from build123d import *

# Parameters (mm, degrees)
SKETCH1_W            = 110
SKETCH1_H            = 58
BOSS_EXTRUDE1_DEPTH  = 4
SKETCH2_R            = 3.398974158
SKETCH2_R_2          = 3.407761536
SKETCH2_R_3          = 1.902710934
SKETCH2_R_4          = 2.384440654
BOSS_EXTRUDE2_DEPTH  = 1.6
BOSS_EXTRUDE3_DEPTH  = 6.2
SKETCH4_R            = 2.45
SKETCH4_R_2          = 1.95
SKETCH4_R_3          = 1.9
SKETCH4_R_4          = 1.2
BOSS_EXTRUDE4_DEPTH  = 4
BOSS_EXTRUDE5_DEPTH  = 1.6
BOSS_EXTRUDE7_DEPTH  = 2
SKETCH10_W           = 9.685953709
SKETCH10_H           = 3.389605022
CUT_EXTRUDE1_DEPTH   = 5
SKETCH11_W           = 9.457855186
SKETCH11_H           = 3.19445865
CUT_EXTRUDE2_DEPTH   = 5
SKETCH12_W           = 7.571734997
SKETCH12_H           = 3.389605022
CUT_EXTRUDE3_DEPTH   = 5
SKETCH13_W           = 8.877658174
SKETCH13_H           = 3.389605022
CUT_EXTRUDE4_DEPTH   = 5
BOSS_EXTRUDE11_DEPTH = 2
SKETCH15_W           = 2.328463334
SKETCH15_H           = 10.356170305
SKETCH15_W_2         = 2.062506364
SKETCH15_H_2         = 9.72645826
SKETCH15_W_3         = 2.09471635
SKETCH15_H_3         = 7.99735701
SKETCH15_W_4         = 2.398553281
CUT_EXTRUDE5_DEPTH   = 10
SKETCH16_R           = 1.5
CUT_EXTRUDE9_DEPTH   = 5


with BuildPart() as part:
    # Sketch1 → Boss-Extrude1 (new body)
    with BuildSketch(Plane(origin=(0, 0, 0), x_dir=(1, 0, 0), z_dir=(0, 1, 0))):
        Rectangle(SKETCH1_W, SKETCH1_H)
    extrude(amount=BOSS_EXTRUDE1_DEPTH)

    # Sketch2 → Boss-Extrude2 (add)
    with BuildSketch(Plane(origin=(0, 4, 0), x_dir=(1, 0, 0), z_dir=(0, 1, 0))):
        Polygon((46.346119795, 25.541263413), (55, 25.541263413), (55, 29), (-54.994341331, 29), (-54.994341331, 25.541263413), (-45.986579734, 25.541263413), (-45.986579734, 18.10232226), (-45.986579734, 17.980527053), (-45.986579734, 16.083408227), (-45.088264615, 15.185093108), (-42.202263878, 15.185093108), (-41.564501972, 15.822855015), (-41.564501972, 18.10232226), (-41.564501972, 25.541263413), (40.304214547, 25.541263413), (41.797555033, 20.604809993), (41.797555033, 16.117567037), (42.441634266, 15.185093108), (45.678891317, 15.185093108), (46.346119795, 16.117567037), align=None)
        with Locations(Location((-13.880988948, 17.14491543, 0), (0, 0, 270))):
            Circle(SKETCH2_R)
        with Locations(Location((20.080301926, 13.55493457, 0), (0, 0, 270))):
            Circle(SKETCH2_R_2)
        with Locations(Location((20.58969132, -10.683370151, 0), (0, 0, 270))):
            Circle(SKETCH2_R_3)
        with Locations(Location((-19.024959871, -10.704463559, 0), (0, 0, 270))):
            Circle(SKETCH2_R_4)
        Polygon((-55, -25.732689432), (-55, -29), (55, -29), (55, -25.732689432), (46.191771323, -25.732689432), (46.191771323, -17.749211072), (41.797555033, -17.720096968), (41.797555033, -25.732689432), (-41.564501972, -25.732689432), (-41.564501972, -19.505766322), (-41.564501972, -16.046735723), (-45.837931694, -16.046735723), (-45.837931694, -19.079806126), (-45.837931694, -25.732689432), (-46.135227773, -25.732689432), align=None)
    extrude(amount=BOSS_EXTRUDE2_DEPTH)

    # Sketch2 → Boss-Extrude3 (add)
    with BuildSketch(Plane(origin=(0, 4, 0), x_dir=(1, 0, 0), z_dir=(0, 1, 0))):
        Polygon((46.346119795, 25.541263413), (55, 25.541263413), (55, 29), (-54.994341331, 29), (-54.994341331, 25.541263413), (-45.986579734, 25.541263413), (-45.986579734, 18.10232226), (-45.986579734, 17.980527053), (-45.986579734, 16.083408227), (-45.088264615, 15.185093108), (-42.202263878, 15.185093108), (-41.564501972, 15.822855015), (-41.564501972, 18.10232226), (-41.564501972, 25.541263413), (40.304214547, 25.541263413), (41.797555033, 20.604809993), (41.797555033, 16.117567037), (42.441634266, 15.185093108), (45.678891317, 15.185093108), (46.346119795, 16.117567037), align=None)
        with Locations(Location((-13.880988948, 17.14491543, 0), (0, 0, 270))):
            Circle(SKETCH2_R)
        with Locations(Location((20.080301926, 13.55493457, 0), (0, 0, 270))):
            Circle(SKETCH2_R_2)
        with Locations(Location((20.58969132, -10.683370151, 0), (0, 0, 270))):
            Circle(SKETCH2_R_3)
        with Locations(Location((-19.024959871, -10.704463559, 0), (0, 0, 270))):
            Circle(SKETCH2_R_4)
        Polygon((-55, -25.732689432), (-55, -29), (55, -29), (55, -25.732689432), (46.191771323, -25.732689432), (46.191771323, -17.749211072), (41.797555033, -17.720096968), (41.797555033, -25.732689432), (-41.564501972, -25.732689432), (-41.564501972, -19.505766322), (-41.564501972, -16.046735723), (-45.837931694, -16.046735723), (-45.837931694, -19.079806126), (-45.837931694, -25.732689432), (-46.135227773, -25.732689432), align=None)
    extrude(amount=BOSS_EXTRUDE3_DEPTH)

    # Sketch4 → Boss-Extrude4 (add)
    with BuildSketch(Plane(origin=(0, 10.2, 0), x_dir=(1, 0, 0), z_dir=(0, 1, 0))):
        with Locations(Location((-13.880988948, 17.14491543, 0), (0, 0, 270))):
            Circle(SKETCH4_R)
        with Locations(Location((20.080301926, 13.55493457, 0), (0, 0, 270))):
            Circle(SKETCH4_R_2)
        with Locations(Location((20.58969132, -10.683370151, 0), (0, 0, 270))):
            Circle(SKETCH4_R_3)
        with Locations(Location((-19.024959871, -10.704463559, 0), (0, 0, 270))):
            Circle(SKETCH4_R_4)
    extrude(amount=BOSS_EXTRUDE4_DEPTH)

    # Sketch5 → Boss-Extrude5 (add)
    with BuildSketch(Plane(origin=(0, 10.2, 0), x_dir=(1, 0, 0), z_dir=(0, 1, 0))):
        Polygon((-54.994341331, 25.541263413), (-54.994341331, 29), (55, 29), (55, 25.541263413), (46.346119795, 25.541263413), (46.346119795, 16.117567037), (45.678891317, 15.185093108), (42.441634266, 15.185093108), (41.797555033, 16.117567037), (41.797555033, 20.604809993), (40.304214547, 25.541263413), (-41.564501972, 25.541263413), (-41.564501972, 18.624421299), (-45.986579734, 18.624421299), (-45.986579734, 25.541263413), align=None)
        Polygon((-55, -29), (-55, -25.732689432), (-45.837931694, -25.732689432), (-45.837931694, -16.046735723), (-41.564501972, -16.046735723), (-41.564501972, -25.732689432), (41.797555033, -25.732689432), (41.797555033, -17.720096968), (46.191771323, -17.749211072), (46.191771323, -25.732689432), (55, -25.732689432), (55, -29), align=None)
    extrude(amount=BOSS_EXTRUDE5_DEPTH)

    # Sketch8 → Boss-Extrude7 (add)
    with BuildSketch(Plane(origin=(0, 11.8, 0), x_dir=(1, 0, 0), z_dir=(0, 1, 0))):
        Polygon((-45.986579734, 25.541263413), (-54.994341331, 25.541263413), (-54.994341331, 29), (55, 29), (55, 25.541263413), (46.346119795, 25.541263413), (46.346119795, 16.117567037), (45.678891317, 15.185093108), (42.441634266, 15.185093108), (41.797555033, 16.117567037), (41.80446192, 16.117567037), (41.80446192, 20.605491868), (41.797555033, 20.604809993), (40.304214547, 25.541263413), (-41.564501972, 25.541263413), (-41.564501972, 24.347016348), (-41.542415728, 24.347016348), (-41.542415728, 18.624421299), (-45.986579734, 18.624421299), align=None)
        Polygon((-55, -29), (-55, -25.732689432), (-45.837931694, -25.732689432), (-45.837931694, -16.046735723), (-41.564501972, -16.046735723), (-41.553155446, -16.046735723), (-41.553155446, -22.919153082), (-41.564501972, -22.919153082), (-41.564501972, -25.732689432), (41.797555033, -25.732689432), (41.797555033, -23.239047925), (41.783488135, -23.239047925), (41.783488135, -19.482944402), (46.191771323, -19.482944402), (46.191771323, -25.732689432), (55, -25.732689432), (55, -29), align=None)
    extrude(amount=BOSS_EXTRUDE7_DEPTH)

    # Sketch10 → Cut-Extrude1 (cut)
    with BuildSketch(Plane.ZY.offset(45.837931694)):
        with Locations((20.889712577, 7.400343861)):
            Rectangle(SKETCH10_W, SKETCH10_H)
    extrude(amount=-CUT_EXTRUDE1_DEPTH, mode=Mode.SUBTRACT)

    # Sketch11 → Cut-Extrude2 (cut)
    with BuildSketch(Plane.ZY.offset(45.986579734)):
        with Locations((-20.81233582, 7.302770675)):
            Rectangle(SKETCH11_W, SKETCH11_H)
    extrude(amount=-CUT_EXTRUDE2_DEPTH, mode=Mode.SUBTRACT)

    # Sketch12 → Cut-Extrude3 (cut)
    with BuildSketch(Plane(origin=(46.191771323, 0, 0), x_dir=(0, 0, -1), z_dir=(1, 0, 0))):
        with Locations((-21.535078571, 7.400343861)):
            Rectangle(SKETCH12_W, SKETCH12_H)
    extrude(amount=-CUT_EXTRUDE3_DEPTH, mode=Mode.SUBTRACT)

    # Sketch13 → Cut-Extrude4 (cut)
    with BuildSketch(Plane(origin=(46.346119795, 0, 0), x_dir=(0, 0, -1), z_dir=(1, 0, 0))):
        with Locations((20.556396124, 7.400343861)):
            Rectangle(SKETCH13_W, SKETCH13_H)
    extrude(amount=-CUT_EXTRUDE4_DEPTH, mode=Mode.SUBTRACT)

    # Sketch14 → Boss-Extrude11 (add)
    with BuildSketch(Plane(origin=(0, 13.8, 0), x_dir=(1, 0, 0), z_dir=(0, 1, 0))):
        Polygon((-55, -25.732689432), (-55, -29), (55, -29), (55, -25.732689432), (46.191771323, -25.732689432), (46.191771323, -19.482944402), (40.796637058, -19.482944402), (40.796637058, -23.53105864), (41.797555033, -23.53105864), (41.797555033, -25.732689432), (-41.564501972, -25.732689432), (-41.564501972, -22.919153082), (-41.558372671, -22.919153082), (-41.553155446, -20.524286948), (-40.212145481, -20.524286948), (-40.212145481, -16.046735723), (-45.837931694, -16.046735723), (-45.837931694, -25.732689432), align=None)
        Polygon((55, 29), (-54.994341331, 29), (-54.994341331, 25.541263413), (-45.986579734, 25.541263413), (-45.986579734, 18.624421299), (-40.393969825, 18.624421299), (-40.393969825, 22.074882647), (-41.564501972, 22.074882647), (-41.564501972, 25.541263413), (40.304214547, 25.541263413), (41.797555033, 20.604809993), (41.797555033, 18.88036778), (40.93151342, 18.88036778), (40.93151342, 15.577482073), (41.797555033, 15.577482073), (41.797555033, 14.916904931), (46.346119795, 14.916904931), (46.346119795, 25.541263413), (55, 25.541263413), align=None)
    extrude(amount=BOSS_EXTRUDE11_DEPTH)

    # Sketch15 → Cut-Extrude5 (cut)
    with BuildSketch(Plane(origin=(0, 15.8, 0), x_dir=(1, 0, 0), z_dir=(0, 1, 0))):
        with Locations((-44.822348067, 20.36317826)):
            Rectangle(SKETCH15_W, SKETCH15_H)
        with Locations((-44.806678512, -20.909964853)):
            Rectangle(SKETCH15_W_2, SKETCH15_H_2)
        with Locations((45.144413148, -21.734010927)):
            Rectangle(SKETCH15_W_3, SKETCH15_H_3)
        with Locations((45.146843155, 20.36317826)):
            Rectangle(SKETCH15_W_4, SKETCH15_H)
    extrude(amount=-CUT_EXTRUDE5_DEPTH, mode=Mode.SUBTRACT)

    # Sketch16 → Cut-Extrude9 (cut)
    with BuildSketch(Plane(origin=(0, 4, 0), x_dir=(1, 0, 0), z_dir=(0, 1, 0))):
        with Locations(Location((-49.750520398, -21.917426264, 0), (0, 0, 270))):
            Circle(SKETCH16_R)
        with Locations(Location((-49.750520398, 21.99224412, 0), (0, 0, 270))):
            Circle(SKETCH16_R)
        with Locations(Location((50.339499411, -21.917426264, 0), (0, 0, 270))):
            Circle(SKETCH16_R)
        with Locations(Location((50.339499411, 21.99224412, 0), (0, 0, 270))):
            Circle(SKETCH16_R)
    extrude(amount=-CUT_EXTRUDE9_DEPTH, mode=Mode.SUBTRACT)


solid = part.part
The model under review builds one solid part; all positions refer to its coordinate system, in mm. A direction names the side the tool comes from. Round coordinates to 2 decimals unless told otherwise and drop trailing zeros. Loops run counter-clockwise (first coordinate to the right, second up) from the corner with the lowest first, then second, coordinate; pieces in that order, holes last. Notation, with made-up numbers: M 9,83.25 L 57,83.25 A18 ccw 57,103.25 Z; hole C -10.5,33.25 d1. An arc over 180 degrees is marked long. Answer as CSV lines item,"result". Start each with the question number.
Item 1: Consider section B-B (z = -5.5). Write out the cut boundary in (x, y), then the cut area to 3 significant figures.
Item 2: Insertion check: P1, Ø4, axis at x = 22.5, z = 15, coming from the +Y side; P2, Ø0.9, axis at y = 5, z = -21, coming from the -X side; P3, Ø5, axis at y = 12.5, z = 16, coming from the -X side. Each pin has a flat end and moves straight along its axis. Give the tip position at first contact, or say it passes through.
Item 3: Wall thickness on line 1 (Y direction, x = -43, z = -23.5); line 2 (Z direction, x = 50, y = 13.5); line 3 (Y direction, x = 43, z = -18): over which ranges is each line inside the solid? List them lowest first. Write a range as [from, to].
Item 4: Consider section C-C (y = 7.75). State how many separate pieces and enclosed holes the cut face has, then the cut area to 3 significant figures.
Item 5: For faces 4 (the face through (43, 7, -16.118)), 5 (the face through (-17.2, 7.06, -17.88)), 6 (the face through (-42, 7, -16.083)), list the 3-axis set-ups (+Z, -Z, +X, -X, +Y, -Y) from which the entire face can be reached by the end or side of a thin tool; tool diameter is ignored.
Item 6: Mouldability with a two-part tool opening along X and no side actions: class faces 1 (the face through (-12, 10.2, -15)), 2 (the face through (43.948, 12, -20)), 3 (the face through (43, 7, 25.321)) as released by +X, released by -X, zero draft, split by the parting line, or undercut.
Item 7: Consider section A-A (x = 36.5). Write out the cut boundary in (y, z).
Answer:
1,outline,"M -55,0 L 55,0 L 55,4 L -55,4 Z"
1,area,"440 mm^2"
2,P1,"stops at y = 4"
2,P2,"stops at x = -45.99"
2,P3,"stops at x = -43.78"
3,line 1,"y = [0, 5.71], [8.9, 15.8]"
3,line 2,"z = [-29, -25.54], [25.73, 29]"
3,line 3,"y = [0, 5.71], [9.1, 15.8]"
4,separate pieces,"9"
4,enclosed holes,"0"
4,area,"849 mm^2"
5,face 4,"+X"
5,face 5,"+Y"
5,face 6,"-X"
6,face 1,"undercut"
6,face 2,"released by +X"
6,face 3,"zero draft"
7,outline,"M 0,-29 L 15.8,-29 L 15.8,-25.54 L 4,-25.54 L 4,25.73 L 15.8,25.73 L 15.8,29 L 0,29 Z"
